Geometry check sheet. Reference: the model listing, model coordinates, mm. A direction names the side the tool comes from. Round coordinates to 2 decimals unless told otherwise and drop trailing zeros. Loops run counter-clockwise (first coordinate to the right, second up) from the corner with the lowest first, then second, coordinate; pieces in that order, holes last. Notation, with made-up numbers: (37.25, 21.5) -> (93.25, 21.5) arc R25 cw to (93.25, 37.5) -> close; hole circle Ø11 at (31.25, -20). An arc over 180 degrees is marked (long way). Use a Markdown table: item, result. Add a question column.
Q1. Gauge pin test, flat ends, axial feed: P1, Ø1, axis at y = 5.5, z = -2.5, coming from the -X side; P2, Ø3, axis at y = 3, z = -2, coming from the +X side. Record the tip position at first contact, or that the pin passes through.
Q2. Sectioned sample at A-A, the plane x = -12. Enter the section's corners in (y, z).
Q3. Sectioned sample at B-B, the plane y = 0. Enter the section's corners in (x, z).
Q4. Material ranges on L1, parallel to Y at x = -115, z = -3.25; L2, parallel to X at y = 8, z = -2; L3, parallel to Y at x = -123.5, z = 3.5, recorded low to high.
Q5. Sectioned sample at C-C, the plane z = -0.75. Enter the section's corners in (x, y).
Q6. Release check for a two-part mould opening along Y. For faces 3 (the face through (-62, 12.22, 0)), 4 (the face through (-66, -11, 4.25)), 5 (the face through (-132.196, -0.235, -0.059)) record: released by +Y, released by -Y, zero draft, split by the parting line, or undercut.
Q7. Set-up check for faces 1 (the face through (-62, 10.7, 0)), 2 (the face through (-133.715, -0.269, -0.059)): record each of +Z, -Z, +X, -X, +Y, -Y from which the full face is reachable in a straight line by a thin tool's end or side.
Autodesk Inventor part; units mm, degrees
ref_plane "YZ Plane" through (0, 0, 0) normal (1, 0, 0) x (0, 1, 0)
ref_plane "XZ Plane" through (0, 0, 0) normal (0, 1, 0) x (-1, 0, 0)
ref_plane "XY Plane" through (0, 0, 0) normal (0, 0, 1) x (1, 0, 0)
sketch "Sketch1" plane through (0, 0, 0) normal (0, 0, 1) x (1, 0, 0)
  arc A0 (0, -11.4595) -> (0, 11.4595) centre (0, 0) ccw construction
  arc A1 (-121.4989, 11.4595) -> (-121.4989, -11.4595) centre (-121.4989, 0) ccw construction
  line L0 (0, -11.4595) -> (-121.4989, -11.4595) construction
  line L1 (0, 11.4595) -> (-121.4989, 11.4595) construction
  dimension "Belt_Teeth" = 105
  dimension "Belt_Pitch2" = 3
  dimension "d0" = 22.919
  dimension "d1" = 22.919
  dimension "d2" = 36.0011
  dimension "d3" = 36.0011
  dimension "Center_Distance" = 121.4989
  dimension "d5" = 121.4989
sketch "Sketch2" plane through (0, 0, 0) normal (0, 0, 1) x (1, 0, 0)
  line L0 (35.7235, 34.2567) -> (38.7235, 34.2567)
  point P0 (0, 0)
  dimension "Belt_Pitch2" = 3
sketch "Sketch4" plane through (0, 0, 0) normal (0, 0, 1) x (1, 0, 0)
  line L0 (-16.1422, -21.869) -> (-14.1422, -21.869)
  line L1 (-16.1422, -21.869) -> (-16.1422, -20.349)
  arc A0 (-15.5872, -20.904) -> (-16.1422, -20.349) centre (-16.1422, -20.904) ccw
  line L2 (-15.5872, -20.904) -> (-15.5872, -20.959)
  arc A1 (-15.5872, -20.959) -> (-15.4372, -21.109) centre (-15.4372, -20.959) ccw
  line L3 (-15.4372, -21.109) -> (-14.8472, -21.109)
  line L4 (-14.1422, -21.869) -> (-14.1422, -20.349)
  arc A2 (-14.1422, -20.349) -> (-14.6972, -20.904) centre (-14.1422, -20.904) ccw
  arc A3 (-14.8472, -21.109) -> (-14.6972, -20.959) centre (-14.8472, -20.959) ccw
  line L5 (-14.6972, -20.959) -> (-14.6972, -20.904)
  line L6 (0, 11.4595) -> (-121.4989, 11.4595) construction
  arc A4 (-121.4989, 11.4595) -> (-121.4989, -11.4595) centre (-121.4989, 0) ccw construction
  line L7 (0, -11.4595) -> (-121.4989, -11.4595) construction
  arc A5 (0, -11.4595) -> (0, 11.4595) centre (0, 0) ccw construction
  arc A6 (-121.4989, 12.2195) -> (-121.4989, -12.2195) centre (-121.4989, 0) ccw
  line L8 (-121.4989, 12.2195) -> (0, 12.2195)
  arc A7 (0, -12.2195) -> (0, 12.2195) centre (0, 0) ccw
  line L9 (0, -12.2195) -> (-121.4989, -12.2195)
  arc A8 (-121.4989, 10.6995) -> (-121.4989, -10.6995) centre (-121.4989, 0) ccw
  line L10 (-121.4989, 10.6995) -> (0, 10.6995)
  arc A9 (0, -10.6995) -> (0, 10.6995) centre (0, 0) ccw
  line L11 (0, -10.6995) -> (-121.4989, -10.6995)
  point P0 (-15.1422, -21.109)
  point P1 (-15.1422, -21.869)
  dimension "d9" = 2
  dimension "d10" = 1.52
  dimension "d11" = 0.76
  dimension "d12" = 0.555
  dimension "d13" = 0.555
  dimension "d14" = 0.15
  dimension "d15" = 0.15
  dimension "belt_thickness" = 1.52
  dimension "d44" = 0.76
extrude "Extrusion2" add sketch "Sketch4" along normal mid plane 8.5 contours L8 A7 L9 A6
sketch "Sketch5" plane through (0, 0, 4.25) normal (0, 0, 1) x (1, 0, 0)
  line L0 (-121.4989, 10.6995) -> (0, 10.6995) construction
  arc A0 (0, -10.6995) -> (0, 10.6995) centre (0, 0) ccw construction
  line L1 (0, -10.6995) -> (-121.4989, -10.6995) construction
  arc A1 (-121.4989, 10.6995) -> (-121.4989, -10.6995) centre (-121.4989, 0) ccw construction
  arc A2 (-121.4989, 12.2195) -> (-121.4989, -12.2195) centre (-121.4989, 0) ccw construction
  line L2 (-121.4989, -12.2195) -> (0, -12.2195) construction
  arc A3 (0, -12.2195) -> (0, 12.2195) centre (0, 0) ccw construction
  line L3 (0, 12.2195) -> (-121.4989, 12.2195) construction
  line L4 (-7.7556, -2.6989) -> (-5.7556, -2.6989)
  line L5 (-7.7556, -2.6989) -> (-7.7556, -1.1789) construction
  arc A4 (-7.2006, -1.7339) -> (-7.7556, -1.1789) centre (-7.7556, -1.7339) ccw
  line L6 (-7.2006, -1.7339) -> (-7.2006, -1.7889)
  arc A5 (-7.2006, -1.7889) -> (-7.0506, -1.9389) centre (-7.0506, -1.7889) ccw
  line L7 (-7.0506, -1.9389) -> (-6.4606, -1.9389)
  line L8 (-5.7556, -2.6989) -> (-5.7556, -1.1789)
  arc A6 (-5.7556, -1.1789) -> (-6.3106, -1.7339) centre (-5.7556, -1.7339) ccw
  arc A7 (-6.4606, -1.9389) -> (-6.3106, -1.7889) centre (-6.4606, -1.7889) ccw
  line L9 (-6.3106, -1.7889) -> (-6.3106, -1.7339)
  line L10 (-8.3106, -1.7339) -> (-8.3106, -1.7889)
  arc A8 (-7.7556, -1.1789) -> (-8.3106, -1.7339) centre (-7.7556, -1.7339) ccw
  arc A9 (-8.4606, -1.9389) -> (-8.3106, -1.7889) centre (-8.4606, -1.7889) ccw
  line L11 (-8.4606, -1.9389) -> (-9.0506, -1.9389)
  line L12 (-7.7556, -2.6989) -> (-9.7556, -2.6989)
  line L13 (-9.2006, -1.7889) -> (-9.2006, -1.7339)
  arc A10 (-9.2006, -1.7339) -> (-9.7556, -1.1789) centre (-9.7556, -1.7339) ccw
  line L14 (-9.7556, -2.6989) -> (-9.7556, -1.1789)
  arc A11 (-9.2006, -1.7889) -> (-9.0506, -1.9389) centre (-9.0506, -1.7889) ccw
  line L15 (-17.66, -0.8495) -> (-14.922, -0.8495) construction
  line L16 (-14.922, -0.8495) -> (-14.922, -2.3671) construction
  line L17 (-14.922, -2.3671) -> (-17.66, -2.3671) construction
  line L18 (-17.66, -2.3671) -> (-17.66, -0.8495) construction
  arc A12 (-15.6383, -1.7102) -> (-16.7483, -1.7102) centre (-16.1933, -1.7102) ccw construction
  line L19 (-16.7483, -1.7102) -> (-16.7483, -1.7652) construction
  arc A13 (-16.8983, -1.9152) -> (-16.7483, -1.7652) centre (-16.8983, -1.7652) ccw construction
  line L20 (-16.7483, -1.7102) -> (-16.7483, -1.9152) construction
  line L21 (-15.6383, -1.7102) -> (-15.6383, -1.9152) construction
  point P0 (-6.7556, -1.9389)
  point P1 (-6.7556, -2.6989)
  point P2 (-8.7556, -2.6989)
  point P3 (-8.7556, -1.9389)
  dimension "d22" = 2
  dimension "d23" = 1.52
  dimension "d24" = 0.76
  dimension "d25" = 0.555
  dimension "d26" = 0.555
  dimension "d27" = 0.15
  dimension "d28" = 0.15
  dimension "d29" = 0.76
  dimension "d30" = 1
  dimension "d31" = 2
  dimension "d32" = 0.59
  dimension "d34" = 0.555
  dimension "d35" = 0
  dimension "d36" = 0
  dimension "d37" = 0.15
  dimension "d38" = 0.055
  dimension "d39" = 0.055
  dimension "d40" = 0
  dimension "d41" = 0
  dimension "d42" = 0.205
  dimension "d43" = 0.205
equation "\"d13\" = d12"
equation "\"d15\" = d14"
equation "\"d44\" = 0.5 * belt_thickness"
equation "\"d26\" = d25"
equation "\"d28\" = d27"
equation "\"d31\" = d22"
equation "\"d43\" = d42"
equation "\"Belt_Teeth\" = 105"
equation "\"Belt_Pitch\" = 3"
equation "\"HTD_5mm\" = 5"
equation "\"GT2_3mm\" = 3"
equation "\"Center_Distance_Copy\" = Center_Distance"
properties part number "GT2-105T" material "Rubber"
Values:
| question | item | result |
|---|---|---|
| 1 | P1 | x = -132.65 |
| 1 | P2 | x = 12.13 |
| 2 | outline | (-12.22, -4.25) -> (-10.7, -4.25) -> (-10.7, 4.25) -> (-12.22, 4.25) -> close; (10.7, -4.25) -> (12.22, -4.25) -> (12.22, 4.25) -> (10.7, 4.25) -> close |
| 3 | outline | (-133.72, -4.25) -> (-132.2, -4.25) -> (-132.2, 4.25) -> (-133.72, 4.25) -> close; (10.7, -4.25) -> (12.22, -4.25) -> (12.22, 4.25) -> (10.7, 4.25) -> close |
| 4 | L1 | -12.22 to -10.7, 10.7 to 12.22 |
| 4 | L2 | -130.74 to -128.6, 7.1 to 9.24 |
| 4 | L3 | -12.05 to -10.51, 10.51 to 12.05 |
| 5 | outline | (-121.5, -12.22) -> (0, -12.22) arc R12.22 ccw to (0, 12.22) -> (-121.5, 12.22) arc R12.22 ccw to start; hole (-121.5, -10.7) -> (0, -10.7) arc R10.7 ccw to (0, 10.7) -> (-121.5, 10.7) arc R10.7 ccw to start |
| 6 | face 3 | released by +Y |
| 6 | face 4 | zero draft |
| 6 | face 5 | undercut |
| 7 | face 1 | +Z, -Z |
| 7 | face 2 | +Z, -Z, -X |
